from build123d import *

# Parameters (mm, degrees)
SKETCH1_R           = 2.15265
SKETCH1_R_2         = 2.487009827
SKETCH1_R_3         = 2.39450721
BOSS_EXTRUDE1_DEPTH = 10.8
SKETCH3_R           = 6.6675
SKETCH3_R_2         = 5.334
CUT_EXTRUDE1_DEPTH  = 7.5


with BuildPart() as part:
    # Sketch1 → Boss-Extrude1 (new body)
    with BuildSketch(Plane.XY):
        with BuildLine():
            Line((0, -17.78), (-45.72, -17.78))
            Line((-45.72, -17.78), (-45.72, -84.1375))
            ThreePointArc((-45.72, -84.1375), (-30.833523511, -114.746148224), (-9.525, -141.2875))
            Line((-9.525, -141.2875), (0, -141.2875))
            Line((0, -141.2875), (0, -17.78))
        make_face()
        with Locations((-36.1315, -33.274)):
            Circle(SKETCH1_R, mode=Mode.SUBTRACT)
        with Locations((-29.5275, -88.7095)):
            Circle(SKETCH1_R, mode=Mode.SUBTRACT)
        with Locations((-9.144, -122.9995)):
            Circle(SKETCH1_R, mode=Mode.SUBTRACT)
        with Locations((-4.3173518, -98.035919174)):
            Circle(SKETCH1_R_2, mode=Mode.SUBTRACT)
        with Locations((-21.024674116, -114.680376144)):
            Circle(SKETCH1_R_3, mode=Mode.SUBTRACT)
        with BuildLine():
            Line((-30.5943, -46.501483685), (-43.185677441, -46.501483685))
            ThreePointArc((-43.185677441, -46.501483685), (-44.308209457, -46.96645167), (-44.773177441, -48.088983685))
            Line((-44.773177441, -48.088983685), (-44.773177441, -78.965225138))
            ThreePointArc((-44.773177441, -78.965225138), (-44.308209457, -80.087757153), (-43.185677441, -80.552725138))
            Line((-43.185677441, -80.552725138), (-18.474223541, -80.552725138))
            ThreePointArc((-18.474223541, -80.552725138), (-17.351691526, -81.017693123), (-16.886723541, -82.140225138))
            Line((-16.886723541, -82.140225138), (-16.886723541, -83.937143103))
            ThreePointArc((-16.886723541, -83.937143103), (-16.421755557, -85.059675118), (-15.299223541, -85.524643103))
            Line((-15.299223541, -85.524643103), (-5.327492268, -85.524643103))
            ThreePointArc((-5.327492268, -85.524643103), (-4.204960252, -85.059675118), (-3.739992268, -83.937143103))
            Line((-3.739992268, -83.937143103), (-3.739992268, -58.7502))
            ThreePointArc((-3.739992268, -58.7502), (-4.204960252, -57.627667985), (-5.327492268, -57.1627))
            Line((-5.327492268, -57.1627), (-6.8707, -57.1627))
            ThreePointArc((-6.8707, -57.1627), (-7.993232015, -56.697732015), (-8.4582, -55.5752))
            Line((-8.4582, -55.5752), (-8.4582, -26.6573))
            ThreePointArc((-8.4582, -26.6573), (-9.053359021, -25.220459021), (-10.4902, -24.6253))
            Line((-10.4902, -24.6253), (-26.9748, -24.6253))
            ThreePointArc((-26.9748, -24.6253), (-28.411640979, -25.220459021), (-29.0068, -26.6573))
            Line((-29.0068, -26.6573), (-29.0068, -44.913983685))
            ThreePointArc((-29.0068, -44.913983685), (-29.471767985, -46.036515701), (-30.5943, -46.501483685))
        make_face(mode=Mode.SUBTRACT)
    extrude(amount=BOSS_EXTRUDE1_DEPTH)

    # Sketch3 → Cut-Extrude1 (cut)
    with BuildSketch(Plane.XY.offset(10.8)):
        with Locations((-9.144, -122.9995)):
            Circle(SKETCH3_R)
        with Locations((-29.5275, -88.7095)):
            Circle(SKETCH3_R)
        with Locations((-36.1315, -33.274)):
            Circle(SKETCH3_R_2)
    extrude(amount=-CUT_EXTRUDE1_DEPTH, mode=Mode.SUBTRACT)


solid = part.part
Design review of the part built by this model. Coordinates are the model's own, in mm. A direction names the side the tool comes from. Give positions to 0.01 mm unless a question says otherwise; leave off trailing zeros. Write each loop counter-clockwise with the first axis right and the second up, starting at its lowest first coordinate (ties: lowest second). Pieces come first, ordered by that corner, then holes. Notation, with made-up numbers: M 68.25,40 L 98.25,40 A34 cw 98.25,77 Z; hole C 78,39.5 d5. An arc over 180 degrees is marked long. Answer as a JSON object with one key per item and string values. Group by question number.
1) Mouldability with a two-part tool opening along Y and no side actions: class faces 4 (the face through (-31.09, -114.34, 5.32)), 5 (the face through (-11, -121, 3.3)), 6 (the face through (-3, -79, 0)) as released by +Y, released by -Y, zero draft, split by the parting line, or undercut.
2) Tool access review of faces 1 (the face through (-8.458, -41, 5)), 2 (the face through (-27, -89, 3.3)), 3 (the face through (-45.72, -50, 5)): name each direction out of +Z, -Z, +X, -X, +Y, -Y from which nothing blocks a thin tool from reaching the whole face with its end or side.
3) Clearance check with flat-ended pins moving along their axes: pin 1 Ø15.5 at (x, y) = (-9.14, -123) entering from +Z; pin 2 Ø4 at (x, y) = (-28.5, -90.5) entering from +Z; pin 3 Ø3 at (x, z) = (-37, 7) entering from -Y; pin 4 Ø5.5 at (x, z) = (-36.5, 7) entering from -Y. State where each tip first meets the part, or that it passes through.
4) We need section B-B (z = 6.75). Count the separate pieces of the cut face and the enclosed holes in it, and give its area (3 significant figures).
5) For line 1 along X through (y, z) = (-54, 5.5); line 2 along X through (y, z) = (-74.5, 9); line 3 along Y through (x, z) = (-34, 5.5), list the stretches that pass through material, from the lowest coordinate up.
6) We need section A-A (y = -69.5). Give the boundary of the cut face in (x, z).
Answer key:
{
 "1": {"face 4": "released by -Y", "face 5": "undercut", "face 6": "zero draft"},
 "2": {"face 1": "+Z, -Z", "face 2": "+Z", "face 3": "+Z, -Z, -X, +Y, -Y"},
 "3": {"pin 1": "stops at z = 10.8", "pin 2": "stops at z = 3.3", "pin 3": "stops at y = -106.86", "pin 4": "stops at y = -109.95"},
 "4": {"separate pieces": "1", "enclosed holes": "6", "area": "2,520 mm²"},
 "5": {"line 1": "x = -45.72 to -44.77, -8.46 to 0", "line 2": "x = -45.72 to -44.77, -3.74 to 0", "line 3": "y = -109.52 to -93.65, -83.76 to -80.55, -46.5 to -38.16, -28.38 to -17.78"},
 "6": {"outline": "M -45.72,0 L -44.77,0 L -44.77,10.8 L -45.72,10.8 Z; M -3.74,0 L 0,0 L 0,10.8 L -3.74,10.8 Z"}
}
